```python
from build123d import *

# Parameters (mm, degrees)
ESQUISSE1_R                 = 22.5
BOSS_EXTRU_1_DEPTH          = 4
ESQUISSE2_R                 = 22.5
ESQUISSE2_R_2               = 21
BOSS_EXTRU_2_DEPTH          = 70
ENL_V_START                 = 20.75783225
ENL_V_MAT_EXTRU_1_OUTLINE_R = 3.18
ENL_V_MAT_EXTRU_1_DEPTH     = 1.742167853


# Read off the part's stored shape, not the designer's step: Enlèv. mat.-Extru.1
with BuildPart() as part:
    # Esquisse1 → Boss.-Extru.1 (new body)
    with BuildSketch(Plane.XY):
        Circle(ESQUISSE1_R)
    extrude(amount=BOSS_EXTRU_1_DEPTH)

    # Esquisse2 → Boss.-Extru.2 (add)
    with BuildSketch(Plane.XY.offset(4)):
        Circle(ESQUISSE2_R)
        Circle(ESQUISSE2_R_2, mode=Mode.SUBTRACT)
    extrude(amount=BOSS_EXTRU_2_DEPTH)

    # Enlèv. mat.-Extru.1 outline → Enlèv. mat.-Extru.1 (cut)
    with BuildSketch(Plane(origin=(0, 0, 0), x_dir=(1, 0, 0), z_dir=(0, 1, 0)).offset(ENL_V_START)):
        with Locations((0, -13.943817021)):
            Circle(ENL_V_MAT_EXTRU_1_OUTLINE_R)
    extrude(amount=ENL_V_MAT_EXTRU_1_DEPTH, mode=Mode.SUBTRACT)


solid = part.part
```
Check sheet for the modelled part. Datum: model origin and axes. Units: mm. A direction names the side the tool comes from. Coordinates: 2 decimals unless noted, no trailing zeros. Order: outer loops, then holes, each group sorted by start corner. A loop starts at its lowest first (then second) coordinate and runs counter-clockwise, first axis right, second up. Notation, with made-up numbers: (20, 39.25) -> (60, 39.25) arc R19 ccw to (60, 74.25) -> close; hole circle Ø10 at (59.5, -4). An arc over 180 degrees is marked (long way). Write each question's results on one line, items separated by ' | '. Start each with the question number.
1) Set-up check for faces 4 (the face through (0, 0, 0)), 5 (the face through (9.69, -18.63, 38.51)), 6 (the face through (3, 22, 15)): record each of +Z, -Z, +X, -X, +Y, -Y from which the full face is reachable in a straight line by a thin tool's end or side.
2) Depth check by flat-ended pin: pin 1 (2 mm diameter, centred on y = 16.5, z = 45, fed in from +X); pin 2 (4 mm diameter, centred on x = 8, z = 22.5, fed in from -Y); pin 3 (6 mm diameter, centred on x = -10.5, z = 33, fed in from -Y). Enter the tip coordinate at first touch or a pass-through.
3) Section check A-A (x = 0). Enter the section's corners in (y, z), and give its area (3 significant figures).
4) Material ranges on line 1 along Z through (x, y) = (0, 22.05); line 2 along Y through (x, z) = (0, 30); line 3 along Z through (x, y) = (-16, 12), recorded low to high.
5) Section check D-D (x = -9.5). Enter the section's corners in (y, z), and give its area (3 significant figures).
6) Section check B-B (y = 0). Enter the section's corners in (x, z), and give its area (3 significant figures).
7) Draft check along Y on faces 1 (the face through (-7, -20, 74)), 2 (the face through (10.382, -19.961, 36.482)), 3 (the face through (0, 0, 4)). Enter one of: pulls with the +Y half, pulls with the -Y half, needs draft (parallel to the pull), parting line crosses it, or undercut.
8) Section check C-C (z = 22). Enter the section's corners in (x, y), and give its area (3 significant figures).
Checked values:
1) face 4: -Z, +X, -X, +Y, -Y | face 5: +Z | face 6: +Y
2) pin 1: x = 16.31 | pin 2: y = -21.69 | pin 3: y = -21.21
3) outline: (-22.5, 0) -> (22.5, 0) -> (22.5, 10.76) -> (21, 10.76) -> (21, 4) -> (-21, 4) -> (-21, 74) -> (-22.5, 74) -> close; (21, 17.12) -> (22.5, 17.12) -> (22.5, 74) -> (21, 74) -> close | area: 380 mm²
4) line 1: 0 to 10.76, 17.12 to 74 | line 2: -22.5 to -21, 21 to 22.5 | line 3: 0 to 4
5) outline: (-20.4, 0) -> (20.4, 0) -> (20.4, 74) -> (18.73, 74) -> (18.73, 4) -> (-18.73, 4) -> (-18.73, 74) -> (-20.4, 74) -> close | area: 397 mm²
6) outline: (-22.5, 0) -> (22.5, 0) -> (22.5, 74) -> (21, 74) -> (21, 4) -> (-21, 4) -> (-21, 74) -> (-22.5, 74) -> close | area: 390 mm²
7) face 1: needs draft | face 2: parting line crosses it | face 3: undercut
8) outline: circle Ø45 at (0, 0); hole circle Ø42 at (0, 0) | area: 205 mm²
